Verification items for the finished model (mm, model axes). A direction names the side the tool comes from. Give positions to 0.01 mm unless a question says otherwise; leave off trailing zeros. Write each loop counter-clockwise with the first axis right and the second up, starting at its lowest first coordinate (ties: lowest second). Pieces come first, ordered by that corner, then holes. Notation, with made-up numbers: (-8.75, 17.5) - (-2.75, 17.5) arc R30 cw to (-2.75, 43.5) - close; hole circle Ø10 at (5, -39). An arc over 180 degrees is marked (long way). Answer as a JSON object with one key per item and string values. Group by question number.
Item 1: Sectioned sample at D-D, the plane z = 45.5. Record the boundary of the cut face in (x, y).
Item 2: Sectioned sample at A-A, the plane z = 6. Record the boundary of the cut face in (x, y).
Item 3: Tool access check on faces 1 (the face through (42.351, -48, 46)), 2 (the face through (-0.24, -10.05, 83.54)), 3 (the face through (33, 40, 86)), 4 (the face through (-62, -35.884, 80)), 5 (the face through (37, -48, 36)). Record the directions out of +Z, -Z, +X, -X, +Y, -Y that give a thin tool (end or side, any length) a straight path to the whole face; none if there is none.
Item 4: Draft check along Z on faces 6 (the face through (6, -45.884, 42)), 7 (the face through (-62.3, -40.95, 77.07)), 8 (the face through (59, -48, 56)). Enter one of: +Z half, -Z half, draft (parallel to the pull), parting line (faces both ways), or undercut.
Item 5: Scan lines: line 1 along Y through (x, z) = (-44.5, 76.5); line 2 along Z through (x, y) = (6, 75). Record each from-to range of solid material in increasing order. Write a range as [from, to].
Item 6: Go/stop test with flat-tipped pins: pin 1 (5.5 mm diameter, centred on y = -48, z = 50.5, fed in from -X); pin 2 (4 mm diameter, centred on x = 63.5, y = -48, fed in from +Z); pin 3 (2 mm diameter, centred on x = 27, z = 41, fed in from +Y); pin 4 (1.5 mm diameter, centred on y = -48, z = 42.5, fed in from +X). Record where each tip stops, or that it passes through.
```python
from build123d import *

# Parameters (mm, degrees)
F0_W     = 150
F0_H     = 140
F1_DEPTH = 86
F2_R     = 3
F3_DEPTH = 10
F2_W     = 30
F2_H     = 20
F2_W_2   = 10
F4_DEPTH = 5
F5_R     = 60
F5_R_2   = 50
F5_R_3   = 45
F5_R_4   = 35
F5_R_5   = 30
F5_R_6   = 15
F5_R_7   = 10
F6_DEPTH = 5
F8_DEPTH = 10


with BuildPart() as f1:
    # F0 (on Top) → F1 (new body)
    with BuildSketch(Plane.XY):
        with Locations((7.351223, 24.116237)):
            Rectangle(F0_W, F0_H)
    extrude(amount=F1_DEPTH)

    # F2 (on face) → F3 (cut)
    with BuildSketch(Plane.XZ.offset(45.883763)):
        with Locations((-61.648777, 80)):
            Circle(F2_R)
        with Locations((-61.648777, 16)):
            Circle(F2_R)
        with Locations((76.351223, 80)):
            Circle(F2_R)
        with Locations((58.351223, 6)):
            Circle(F2_R)
    extrude(amount=-F3_DEPTH, mode=Mode.SUBTRACT)

    # F2 (on face) → F4 (join)
    with BuildSketch(Plane.XZ.offset(45.883763)):
        with Locations((59.351223, 46)):
            Rectangle(F2_W, F2_H)
        with Locations((37.351223, 46)):
            Rectangle(F2_W_2, F2_H)
    extrude(amount=F4_DEPTH)

    # F5 (on face) → F6 (cut)
    with BuildSketch(Plane.XY.offset(86)):
        with Locations((7.351223, 24.116237)):
            Circle(F5_R)
        with Locations((7.351223, 24.116237)):
            Circle(F5_R_2, mode=Mode.SUBTRACT)
        with Locations((7.351223, 24.116237)):
            Circle(F5_R_3)
        with Locations((7.351223, 24.116237)):
            Circle(F5_R_4, mode=Mode.SUBTRACT)
        with Locations((7.351223, 24.116237)):
            Circle(F5_R_5)
        with Locations((7.351223, 24.116237)):
            Circle(F5_R_6, mode=Mode.SUBTRACT)
        with Locations((7.351223, 24.116237)):
            Circle(F5_R_7)
    extrude(amount=-F6_DEPTH, mode=Mode.SUBTRACT)

    # F7 (on face) → F8 (join)
    with BuildSketch(Plane(origin=(0, 94.116237, 0), x_dir=(-1, 0, 0), z_dir=(0, 1, 0))):
        with BuildLine():
            ThreePointArc((-82.351223, 25.255258), (-69.803796, 30.452573), (-64.606481, 43))
            ThreePointArc((-64.606481, 43), (-69.803796, 55.547427), (-82.351223, 60.744742))
            Line((-82.351223, 60.744742), (-82.351223, 25.255258))
        make_face()
    extrude(amount=F8_DEPTH)


solid = f1.part
```
Geometry check:
{
 "1": {"outline": "(-67.65, -45.88) - (32.35, -45.88) - (32.35, -50.88) - (42.35, -50.88) - (42.35, -45.88) - (44.35, -45.88) - (44.35, -50.88) - (74.35, -50.88) - (74.35, -45.88) - (82.35, -45.88) - (82.35, 104.12) - (64.78, 104.12) - (64.78, 94.12) - (-67.65, 94.12) - close"},
 "2": {"outline": "(-67.65, -45.88) - (55.35, -45.88) - (55.35, -35.88) - (61.35, -35.88) - (61.35, -45.88) - (82.35, -45.88) - (82.35, 94.12) - (-67.65, 94.12) - close"},
 "3": {"face 1": "+Z, -Z, -Y", "face 2": "+Z", "face 3": "+Z, +X, -X, +Y, -Y", "face 4": "-Y", "face 5": "-Z, +X, -X, -Y"},
 "4": {"face 6": "draft", "face 7": "undercut", "face 8": "+Z half"},
 "5": {"line 1": "[-45.88, 94.12]", "line 2": "[0, 81]"},
 "6": {"pin 1": "x = -67.65", "pin 2": "z = 56", "pin 3": "y = 94.12", "pin 4": "x = 74.35"}
}
